Work out the finished part from the listing and answer in its coordinate system (mm). Give positions to 0.01 mm unless a question says otherwise; leave off trailing zeros. Loops run counter-clockwise (first coordinate to the right, second up) from the corner with the lowest first, then second, coordinate; pieces in that order, holes last. Notation, with made-up numbers: (-3, -11.75) - (7, -11.75) arc R19 cw to (7, 5.25) - close; hole circle Ø5 at (10.5, 4.25). An arc over 180 degrees is marked (long way). One line per question, with ' | ' between items. Start each with the question number.
1. Find the intervals of material crossed by line 1 (Z direction, x = -9.5, y = 2.1) (3 decimals); line 2 (Z direction, x = 10.5, y = 2.1); line 3 (X direction, y = 0.65, z = 175), in increasing order.
2. Each of these flat-tipped pins is pushed along its axis until it touches: pin 1 (4 mm diameter, centred on x = 0, z = 65.025, fed in from -Y); pin 2 (1 mm diameter, centred on y = 0.5, z = 175.5, fed in from -X). Where does it stop, or does it pass through?
3. Section A-A (y = 2.3) is taken. Determine the outline of the cut face in (x, z) (3 decimals), plus the area to 3 significant figures.
4. Section B-B (x = 38.5) is taken. Determine the outline of the cut face in (y, z) (3 decimals).
5. Section C-C (x = -36) is taken. Determine the outline of the cut face in (y, z) (3 decimals), plus the area to 3 significant figures.
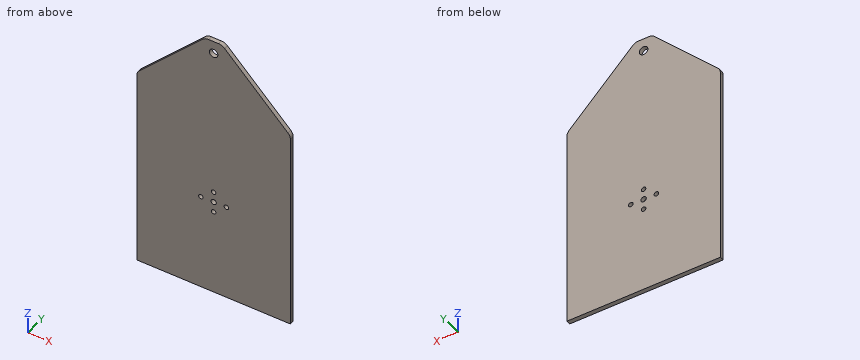
from build123d import *

# Parameters (mm, degrees)
SKETCH1_R               = 3.175
BOSS_EXTRUDE1_DEPTH     = 3.175
CUT_EXTRUDE1_REACH      = 213.108
SKETCH2_R               = 2
ADVANCEDHOLE1_OUTLINE_R = 1.7
ADVANCEDHOLE1_DEPTH     = 3.175


# Read off the part's stored shape, not the designer's step: AdvancedHole1
with BuildPart() as part:
    # Sketch1 → Boss-Extrude1 (new body)
    with BuildSketch(Plane(origin=(0, 0, 0), x_dir=(1, 0, 0), z_dir=(0, 1, 0))):
        with BuildLine():
            Line((-57.15, 0), (57.15, 0))
            Line((57.15, 0), (57.15, -149.769743879))
            ThreePointArc((57.15, -149.769743879), (56.666635031, -152.199783674), (55.290128061, -154.259871939))
            Line((55.290128061, -154.259871939), (8.209871939, -201.340128061))
            ThreePointArc((8.209871939, -201.340128061), (6.149783674, -202.716635031), (3.719743879, -203.2))
            Line((3.719743879, -203.2), (-3.719743879, -203.2))
            ThreePointArc((-3.719743879, -203.2), (-6.149783674, -202.716635031), (-8.209871939, -201.340128061))
            Line((-8.209871939, -201.340128061), (-55.290128061, -154.259871939))
            ThreePointArc((-55.290128061, -154.259871939), (-56.666635031, -152.199783674), (-57.15, -149.769743879))
            Line((-57.15, -149.769743879), (-57.15, 0))
        make_face()
        with Locations(Location((0, -193.675, 0), (0, 0, 270))):
            Circle(SKETCH1_R, mode=Mode.SUBTRACT)
    extrude(amount=BOSS_EXTRUDE1_DEPTH)

    # Sketch2 → Cut-Extrude1 (cut, up to next)
    with BuildSketch(Plane(origin=(0, 3.175, 0), x_dir=(1, 0, 0), z_dir=(0, 1, 0)), mode=Mode.PRIVATE) as cut_extrude1_sk1:
        with Locations(Location((0, -73.025, 0), (0, 0, 270))):
            Circle(SKETCH2_R)
    cut_extrude1_tool1 = extrude(cut_extrude1_sk1.sketch, amount=-CUT_EXTRUDE1_REACH, mode=Mode.PRIVATE) & part.part
    add(cut_extrude1_tool1.solids().sort_by_distance((0, 3.175, 73.025))[0], mode=Mode.SUBTRACT)

    # AdvancedHole1 outline → AdvancedHole1 (cut)
    with BuildSketch(Plane(origin=(0, 0, 0), x_dir=(1, 0, 0), z_dir=(0, 1, 0))):
        with Locations((9.5, -73.025)):
            Circle(ADVANCEDHOLE1_OUTLINE_R)
        with Locations((0, -81.025)):
            Circle(ADVANCEDHOLE1_OUTLINE_R)
        with Locations((-9.5, -73.025)):
            Circle(ADVANCEDHOLE1_OUTLINE_R)
        with Locations((0, -65.025)):
            Circle(ADVANCEDHOLE1_OUTLINE_R)
    extrude(amount=ADVANCEDHOLE1_DEPTH, mode=Mode.SUBTRACT)


solid = part.part
Conclusion:
1) line 1: 0 to 71.325, 74.725 to 200.05 | line 2: 0 to 71.65, 74.4 to 199.05 | line 3: -34.55 to 34.55
2) pin 1: y = 0 | pin 2: x = -34.55
3) outline: (-57.15, 0) - (57.15, 0) - (57.15, 149.77) arc R6.35 ccw to (55.29, 154.26) - (8.21, 201.34) arc R6.35 ccw to (3.72, 203.2) - (-3.72, 203.2) arc R6.35 ccw to (-8.21, 201.34) - (-55.29, 154.26) arc R6.35 ccw to (-57.15, 149.77) - close; hole circle Ø3.4 at (-9.5, 73.025); hole circle Ø6.35 at (0, 193.675); hole circle Ø4 at (0, 73.025); hole circle Ø3.4 at (0, 65.025); hole circle Ø3.4 at (0, 81.025); hole circle Ø3.4 at (9.5, 73.025) | area: 20,600 mm²
4) outline: (0, 0) - (3.175, 0) - (3.175, 171.05) - (0, 171.05) - close
5) outline: (0, 0) - (3.175, 0) - (3.175, 173.55) - (0, 173.55) - close | area: 551 mm²
